Autodesk Inventor part; units mm, degrees
ref_plane "YZ Plane" through (0, 0, 0) normal (1, 0, 0) x (0, 1, 0)
ref_plane "XZ Plane" through (0, 0, 0) normal (0, 1, 0) x (-1, 0, 0)
ref_plane "XY Plane" through (0, 0, 0) normal (0, 0, 1) x (1, 0, 0)
sketch "Boceto1" plane through (0, 0, 0) normal (0, 1, 0) x (-1, 0, 0)
  line L0 (0, 0) -> (-530, 0)
  line L1 (-530, 0) -> (-530, -600)
  line L2 (-530, -600) -> (0, -600)
  line L3 (0, -600) -> (0, 0)
  dimension "d0" = 530
  dimension "d1" = 600
extrude "Extrusión1" add sketch "Boceto1" along normal blind 840
sketch "Boceto2" plane through (530, 0, 0) normal (1, 0, 0) x (0, 0, -1)
  line L0 (0, 0) -> (0, 840)
  line L1 (0, 840) -> (10, 840)
  line L2 (10, 840) -> (10, 830)
  line L3 (10, 830) -> (0, 830)
  line L4 (0, 830) -> (0, 840)
  line L5 (10, 830) -> (590, 830)
  line L6 (590, 830) -> (590, 10)
  line L7 (590, 10) -> (10, 10)
  line L8 (10, 10) -> (10, 830)
  dimension "d4" = 10
  dimension "d5" = 10
  dimension "d6" = 580
  dimension "d7" = 820
extrude "Extrusión2" cut sketch "Boceto2" against normal blind 520 contours L5 L6 L7 L8
sketch "Boceto3" plane through (0, 0, 0) normal (0, 0, 1) x (1, 0, 0)
  line L0 (530, 830) -> (10, 830)
  line L1 (10, 830) -> (520, 830) construction
  line L2 (520, 830) -> (520, 580) construction
  line L3 (520, 580) -> (10, 580) construction
  line L4 (10, 580) -> (10, 830) construction
  line L5 (265, 830) -> (265, 580) construction
  line L6 (265, 580) -> (265, 640)
  line L7 (265, 640) -> (290, 640) construction
  line L8 (265, 640) -> (240, 640) construction
  line L9 (290, 640) -> (302.5, 640) construction
  line L10 (240, 640) -> (227.5, 640) construction
  circle A0 centre (302.5, 640) radius 12.5
  circle A1 centre (227.5, 640) radius 12.5
  line L11 (227.5, 640) -> (227.5, 710) construction
  line L12 (302.5, 640) -> (302.5, 710) construction
  circle A2 centre (227.5, 710) radius 12.5
  circle A3 centre (302.5, 710) radius 12.5
  line L13 (10, 830) -> (10, 10) construction
  line L14 (10, 830) -> (10, 705) construction
  point P0 (0, 0)
  dimension "d10" = 510
  dimension "d11" = 250
  dimension "d12" = 255
  dimension "d13" = 0
  dimension "d14" = 60
  dimension "d15" = 25
  dimension "d16" = 25
  dimension "d17" = 12.5
  dimension "d18" = 12.5
  dimension "d19" = 70
  dimension "d20" = 70
  dimension "d21" = 25
  dimension "d22" = 25
  dimension "d23" = 125
extrude "Extrusión3" add sketch "Boceto3" along normal blind 10
sketch "Boceto4" plane through (302.5, 710, 10) normal (0, 0, 1) x (1, 0, 0)
  circle A0 centre (0, 0) radius 11.5
  circle A1 centre (-75, 0) radius 12.5
  circle A2 centre (-75, 0) radius 11.5
  circle A3 centre (-75, 0) radius 12.5
  circle A4 centre (0, -70) radius 12.5
  circle A5 centre (-75, 0) radius 12.5
  circle A6 centre (-75, -70) radius 12.5
  circle A7 centre (0, 0) radius 12.5
  line L0 (-302.5, -710) -> (227.5, -710)
  line L1 (227.5, -710) -> (227.5, 130)
  line L2 (-302.5, 130) -> (227.5, 130)
  line L3 (-302.5, -710) -> (-302.5, 130)
  line L4 (-302.5, -710) -> (-302.5, 130)
  line L5 (0, 0) -> (-302.5, 0)
  line L6 (-302.5, 0) -> (-302.5, -710)
  line L7 (-302.5, -710) -> (0, -710)
  line L8 (0, -710) -> (0, 0)
  dimension "d26" = 23
  dimension "d27" = 23
  dimension "d29" = 75
  dimension "d30" = 710
  dimension "d31" = 302.5
extrude "Extrusión4" cut sketch "Boceto4" against normal blind 2 contours A0 L8 L5 | L5 L8 A0 | L5 A2 | A2 L5
fillet "Empalme1" radius 3 2 edges at (215, 640, 10) (290, 640, 10)
sketch "Boceto5" plane through (0, 0, 0) normal (0, 0, 1) x (1, 0, 0)
  circle A0 centre (302.5, 640) radius 12.5
  circle A1 centre (227.5, 710) radius 12.5
  circle A2 centre (227.5, 640) radius 12.5
  circle A3 centre (302.5, 710) radius 12.5
  line L0 (0, 0) -> (530, 0)
  line L1 (530, 0) -> (530, 840)
  line L2 (0, 840) -> (530, 840)
  line L3 (0, 0) -> (0, 840)
  line L4 (530, 830) -> (10, 830) construction
  line L5 (10, 830) -> (520, 830) construction
  line L6 (520, 830) -> (520, 630) construction
  line L7 (520, 630) -> (10, 630) construction
  line L8 (10, 630) -> (10, 830) construction
  line L9 (520, 630) -> (435, 630) construction
  line L10 (435, 630) -> (435, 770) construction
  line L11 (10, 630) -> (75, 630) construction
  line L12 (75, 630) -> (75, 770) construction
  line L13 (435, 770) -> (435, 795) construction
  line L14 (435, 795) -> (410, 795) construction
  line L15 (410, 795) -> (460, 795)
  line L16 (460, 795) -> (460, 745)
  line L17 (460, 745) -> (410, 745)
  line L18 (410, 745) -> (410, 795)
  dimension "d35" = 510
  dimension "d36" = 200
  dimension "d37" = 85
  dimension "d38" = 140
  dimension "d39" = 65
  dimension "d40" = 140
  dimension "d41" = 25
  dimension "d42" = 25
  dimension "d43" = 50
  dimension "d44" = 50
extrude "Extrusión5" add sketch "Boceto5" along normal blind 15 contours L15 L16 L17 L18
sketch "Boceto7" plane through (0, 0, 15) normal (0, 0, 1) x (1, 0, 0)
  line L0 (410, 745) -> (460, 745) construction
  line L1 (460, 745) -> (460, 795) construction
  line L2 (460, 795) -> (410, 795) construction
  line L3 (410, 795) -> (410, 745) construction
  line L4 (460, 745) -> (410, 745) construction
  line L5 (410, 745) -> (435, 745) construction
  line L6 (435, 745) -> (435, 770) construction
  line L7 (435, 770) -> (410, 770) construction
  line L8 (410, 770) -> (410, 745) construction
  point P0 (0, 0)
  dimension "d53" = 25
  dimension "d54" = 25
ref_plane "Plano de trabajo1" through (435, 770, 15) normal (-1, 0, 0) x (0, -1, 0)
sketch "Boceto8" plane through (435, 770, 15) normal (-1, 0, 0) x (0, -1, 0)
  line L0 (-25, 0) -> (25, 0) construction
  line L1 (0, 0) -> (0, 50)
  line L2 (0, 0) -> (50, 0) construction
  line L3 (0, 50) -> (-15, 50)
  line L4 (0, 50) -> (15, 50) construction
  line L5 (-15, 50) -> (-15, 40)
  line L6 (0, 0) -> (-10, 0)
  line L7 (-10, 0) -> (-15, 40)
  point P0 (770, -15)
  dimension "d55" = 50
  dimension "d56" = 90
  dimension "d57" = 15
  dimension "d58" = 180
  dimension "d59" = 10
  dimension "d60" = 10
revolve "Revolución1" add sketch "Boceto8" angle 360 about axis through (435, 770, 15) along (0, 0, 1)
fillet "Empalme3" radius 5 1 edges at (435, 755, 65)
fillet "Empalme4" radius 5 1 edges at (435, 760, 15)
sketch "Boceto9" plane through (0, 0, 0) normal (0, 0, 1) x (1, 0, 0)
  line L0 (530, 830) -> (10, 830) construction
  line L1 (10, 830) -> (10, 10) construction
  line L2 (10, 830) -> (520, 830) construction
  line L3 (520, 830) -> (520, 630) construction
  line L4 (520, 630) -> (10, 630) construction
  line L5 (10, 630) -> (10, 830) construction
  line L6 (10, 630) -> (95, 630) construction
  line L7 (95, 630) -> (95, 750) construction
  line L8 (95, 750) -> (10, 750) construction
  line L9 (10, 750) -> (10, 630) construction
  line L10 (95, 750) -> (95, 785) construction
  circle A0 centre (95, 750) radius 35
  point P0 (0, 0)
  dimension "d64" = 510
  dimension "d65" = 200
  dimension "d66" = 85
  dimension "d67" = 120
  dimension "d68" = 35
  dimension "d69" = 70
extrude "Extrusión7" add sketch "Boceto9" along normal blind 10
sketch "Boceto10" plane through (95, 750, 10) normal (0, 0, 1) x (1, 0, 0)
  circle A0 centre (0, 0) radius 30
  line L0 (0, 0) -> (0, 7) construction
  line L1 (0, 0) -> (-5, 0) construction
  line L2 (0, 0) -> (5, 0) construction
  line L3 (0, -30) -> (0, -29.5) construction
  line L4 (0, -29.5) -> (5.454356, -29.5) construction
  line L5 (0, -29.5) -> (-5.454356, -29.5) construction
  line L6 (0, -29.5) -> (-2.727178, -29.5) construction
  line L7 (0, -29.5) -> (2.727178, -29.5) construction
  line L8 (-5, 0) -> (0, 7)
  line L9 (0, 7) -> (5, 0)
  line L10 (2.727178, -29.5) -> (5, 0)
  line L11 (-5, 0) -> (-2.727178, -29.5)
  circle A1 centre (0, 0) radius 35
  circle A2 centre (0, 0) radius 29.625791
  point P0 (-95, -750)
  point P1 (2.727178, -29.5)
  dimension "d72" = 60
  dimension "d73" = 7
  dimension "d74" = 5
  dimension "d75" = 5
  dimension "d76" = 0.5
sketch "Boceto10 outline for Extrusión8" plane through (95, 750, 10) normal (0, 0, 1) x (1, 0, 0)
  line L0 (0, 7) -> (5, 0)
  line L1 (-5, 0) -> (0, 7)
  line L2 (-2.727178, -29.5) -> (-5, 0)
  arc A0 (2.727178, -29.5) -> (-2.727178, -29.5) centre (0, 0) ccw
  line L3 (5, 0) -> (2.727178, -29.5)
extrude "Extrusión8" cut sketch "Boceto10 outline for Extrusión8" against normal blind 9
sketch "Boceto11" plane through (95, 750, 10) normal (0, 0, 1) x (1, 0, 0)
  circle A0 centre (0, 0) radius 33.75
  point P0 (-95, -750)
  dimension "d79" = 67.5
extrude "Extrusión9" cut sketch "Boceto11" against normal blind 2
sketch "Boceto12" plane through (530, 0, 0) normal (1, 0, 0) x (0, 0, -1)
  line L0 (10, 830) -> (590, 830) construction
  line L1 (590, 830) -> (590, 10) construction
  line L2 (590, 10) -> (10, 10) construction
  line L3 (10, 10) -> (10, 830) construction
  line L4 (0, 0) -> (600, 0) construction
  line L5 (600, 0) -> (600, 840) construction
  line L6 (0, 840) -> (600, 840) construction
  line L7 (0, 0) -> (0, 840) construction
  line L8 (600, 0) -> (600, 840) construction
  line L9 (600, 840) -> (600, 720) construction
  line L10 (600, 0) -> (0, 0) construction
  line L11 (600, 0) -> (600, 120) construction
  line L12 (590, 830) -> (590, 10)
  line L13 (600, 120) -> (590, 120)
  line L14 (590, 120) -> (590, 200)
  line L15 (590, 200) -> (600, 200)
  line L16 (600, 200) -> (600, 120)
  line L17 (600, 720) -> (590, 720)
  line L18 (590, 720) -> (590, 640)
  line L19 (590, 640) -> (600, 640)
  line L20 (600, 640) -> (600, 720)
  dimension "d82" = 120
  dimension "d83" = 120
  dimension "d84" = 80
  dimension "d85" = 80
extrude "Extrusión10" add sketch "Boceto12" along normal blind 1
sketch "Boceto13" plane through (531, 0, 0) normal (1, 0, 0) x (0, 0, -1)
  line L0 (600, 0) -> (0, 0)
  line L1 (0, 0) -> (0, 840)
  line L2 (600, 840) -> (0, 840)
  line L3 (600, 0) -> (600, 840)
extrude "Extrusión11" add sketch "Boceto13" along normal blind 9
sketch "Boceto14" plane through (540, 0, 0) normal (1, 0, 0) x (0, 0, -1)
  line L0 (0, 0) -> (600, 0) construction
  line L1 (600, 0) -> (600, 840) construction
  line L2 (600, 840) -> (0, 840) construction
  line L3 (0, 840) -> (0, 0) construction
  line L4 (0, 840) -> (0, 0) construction
  line L5 (0, 840) -> (80, 840) construction
  line L6 (80, 840) -> (80, 760) construction
  line L7 (80, 760) -> (0, 760) construction
  line L8 (0, 760) -> (0, 840) construction
  line L9 (600, 0) -> (520, 0) construction
  line L10 (520, 0) -> (520, 80) construction
  line L11 (520, 80) -> (600, 80) construction
  line L12 (600, 80) -> (600, 0) construction
  line L13 (80, 760) -> (520, 760)
  line L14 (520, 760) -> (520, 80)
  line L15 (520, 80) -> (80, 80)
  line L16 (80, 80) -> (80, 760)
  dimension "d90" = 80
  dimension "d91" = 80
  dimension "d92" = 80
  dimension "d93" = 80
extrude "Extrusión12" cut sketch "Boceto14" against normal blind 8
properties part number "Tablero Maya"
For this review, take the finished solid that the model builds, in its own axes (mm). A direction names the side the tool comes from. Round coordinates to 2 decimals unless told otherwise and drop trailing zeros. Write each loop counter-clockwise with the first axis right and the second up, starting at its lowest first coordinate (ties: lowest second). Pieces come first, ordered by that corner, then holes. Notation, with made-up numbers: M 13,-16.75 L 21,-16.75 A31 ccw 21,13.25 Z; hole C 34.5,38.5 d10. An arc over 180 degrees is marked long. Write item = value, one per line. Start each with the question number.
(1) We need section C-C (y = 376). Give the boundary of the cut face in (x, z).
(2) For faces 1 (the face through (532, 425, -297)), 2 (the face through (232.81, 699.8, 9.01)), 3 (the face through (274, 426, -590)), list the 3-axis set-ups (+Z, -Z, +X, -X, +Y, -Y) from which the entire face can be reached by the end or side of a thin tool; tool diameter is ignored.
(3) We need section A-A (z = -543). Give the boundary of the cut face in (x, y), then the cut area to 3 significant figures.
(4) Clearance check with flat-ended pins moving along their axes: pin 1 Ø6 at (y, z) = (289, -182) entering from +X; pin 2 Ø4.5 at (x, z) = (446.5, 9) entering from -Y; pin 3 Ø7.5 at (x, y) = (227.5, 707.5) entering from +Z; pin 4 Ø1 at (x, z) = (295.5, -509.5) entering from -Y. State where each tip first meets the part, or that it passes through.
(5) We need section D-D (y = 162). Give the boundary of the cut face in (x, z).
(6) For line 1 along X through (y, z) = (710, 8.8); line 2 along Z through (x, y) = (203, 531.5); line 3 along Y through (x, z) = (445.5, -359), list the stretches that pass through material, from the lowest coordinate up.
(7) We need section B-B (x = 275.5). Give the boundary of the cut face in (y, z).
(8) The part is to be moulded in two halves that separate along Z. For faces 4 (the face through (431.131, 782.287, 38.051)), 5 (the face through (233.27, 651.09, 3.45)), 6 (the face through (302, 710, 8)), say which applies: +Z half, -Z half, draft (parallel to the pull), parting line (faces both ways), or undercut.
Results found:
q1.outline = M 0,-600 L 530,-600 L 530,-590 L 10,-590 L 10,-10 L 530,-10 L 530,0 L 0,0 Z; M 531,-600 L 540,-600 L 540,-520 L 532,-520 L 532,-80 L 540,-80 L 540,0 L 531,0 Z
q2.face_1 = +X
q2.face_2 = +Z
q2.face_3 = none
q3.outline = M 0,0 L 530,0 L 530,10 L 10,10 L 10,830 L 530,830 L 530,840 L 0,840 Z; M 531,0 L 540,0 L 540,840 L 531,840 Z
q3.area = 26,400 mm²
q4.pin_1 = 532
q4.pin_2 = 745
q4.pin_3 = 8
q4.pin_4 = 0
q5.outline = M 0,-600 L 540,-600 L 540,-520 L 532,-520 L 532,-80 L 540,-80 L 540,0 L 531,0 L 531,-590 L 10,-590 L 10,-10 L 530,-10 L 530,0 L 0,0 Z
q6.line_1 = 215 to 216, 239 to 240, 290 to 291, 314 to 315
q6.line_2 = -600 to -590, -10 to 0
q6.line_3 = 0 to 10, 830 to 840
q7.outline = M 0,-600 L 840,-600 L 840,0 L 0,0 Z; hole M 10,-590 L 830,-590 L 830,-10 L 10,-10 Z
q8.face_4 = undercut
q8.face_5 = draft
q8.face_6 = +Z half
